Could you check a few things on this model? Use its own coordinates, in mm. A direction names the side the tool comes from. Coordinates: 2 decimals unless noted, no trailing zeros. Write each loop counter-clockwise with the first axis right and the second up, starting at its lowest first coordinate (ties: lowest second). Pieces come first, ordered by that corner, then holes. Notation, with made-up numbers: (-39.75, 23) - (10.25, 23) arc R26 cw to (10.25, 54) - close; hole circle Ø9 at (-34.75, -32). An arc over 180 degrees is marked (long way). Write item = value, one per line. Start each with the question number.
```python
from build123d import *

# Parameters (mm, degrees)
SKETCH1_W           = 147
SKETCH1_H           = 85
BOSS_EXTRUDE1_DEPTH = 57
SKETCH2_W           = 85
SKETCH2_H           = 85
BOSS_EXTRUDE2_DEPTH = 8
SKETCH3_W           = 24
SKETCH3_H           = 31
BOSS_EXTRUDE3_DEPTH = 1


with BuildPart() as part:
    # Sketch1 → Boss-Extrude1 (new body)
    with BuildSketch(Plane.XY):
        Rectangle(SKETCH1_W, SKETCH1_H)
    extrude(amount=BOSS_EXTRUDE1_DEPTH)

    # Sketch2 → Boss-Extrude2 (add)
    with BuildSketch(Plane.XY.offset(57)):
        Rectangle(SKETCH2_W, SKETCH2_H)
    extrude(amount=BOSS_EXTRUDE2_DEPTH)

    # Sketch3 → Boss-Extrude3 (add)
    with BuildSketch(Plane.ZY.offset(73.5)):
        with Locations((42, -20)):
            Rectangle(SKETCH3_W, SKETCH3_H)
    extrude(amount=BOSS_EXTRUDE3_DEPTH)


solid = part.part
```
1) Which directions (+Z, -Z, +X, -X, +Y, -Y) give clear straight access to the entire face, cutting with the end or side of a thin tool? Please do faces 1 (the flat face through (42.5, -1, 61)), 2 (the flat face through (-58, 1, 57)), 3 (the flat face through (-74.5, -20, 42)).
2) Suppose I cut it at C-C on y = 29.5. Please give me the cut outline in (x, z), plus the area to 3 significant figures.
3) Suppose I cut it at A-A on y = -12. Please give me the cut outline in (x, z), plus the area to 3 significant figures.
4) For P1, Ø1.1, axis at x = -74, z = 47, coming from the +Y side; P2, Ø1.5, axis at x = -57, y = 22, coming from the +Z side; P3, Ø6.5, axis at y = 13.5, z = 59.5, coming from the -X side; P4, Ø4, axis at y = -15.5, z = 61, coming from the +X side, each with a flat end and sliding along its axis, tell me the tip position at first contact or that it passes through.
5) Suppose I cut it at B-B on x = 56. Please give me the cut outline in (y, z).
6) If I drill on probe 1 along X at (y, z) = (6, 11); probe 2 along Z at (x, y) = (-54, -23); probe 3 along X at (y, z) = (23, 61), over which ranges is the centre line in solid material (lowest first)? Write a range as [from, to].
Reply:
q1.face_1 = +Z, +X, +Y, -Y
q1.face_2 = +Z, -X, +Y, -Y
q1.face_3 = +Z, -Z, -X, +Y, -Y
q2.outline = (-73.5, 0) - (73.5, 0) - (73.5, 57) - (42.5, 57) - (42.5, 65) - (-42.5, 65) - (-42.5, 57) - (-73.5, 57) - close
q2.area = 9,060 mm^2
q3.outline = (-74.5, 30) - (-73.5, 30) - (-73.5, 0) - (73.5, 0) - (73.5, 57) - (42.5, 57) - (42.5, 65) - (-42.5, 65) - (-42.5, 57) - (-73.5, 57) - (-73.5, 54) - (-74.5, 54) - close
q3.area = 9,080 mm^2
q4.P1 = 42.5
q4.P2 = 57
q4.P3 = -73.5
q4.P4 = 42.5
q5.outline = (-42.5, 0) - (42.5, 0) - (42.5, 57) - (-42.5, 57) - close
q6.probe_1 = [-73.5, 73.5]
q6.probe_2 = [0, 57]
q6.probe_3 = [-42.5, 42.5]
